Source: CAD feature listing. Evaluate the final solid. Frame: model axes, mm. A direction names the side the tool comes from. Give positions to 0.01 mm unless a question says otherwise; leave off trailing zeros. Order: outer loops, then holes, each group sorted by start corner. A loop starts at its lowest first (then second) coordinate and runs counter-clockwise, first axis right, second up.
```python
from build123d import *

# Parameters (mm, degrees)
PAD_DEPTH    = 0.375
SKETCH002_R  = 1.5
PAD001_DEPTH = 0.5


with BuildPart() as part:
    # Sketch → Pad (new body, symmetric)
    with BuildSketch(Plane.XY):
        with BuildLine():
            Line((-0.25, 0), (0, 0))
            Line((0, 0), (0.25, 0))
            ThreePointArc((0.25, 0), (8.71609, -20.785997), (29.295895, -29.741667))
            ThreePointArc((29.290002, -30.241667), (30.749948, -30.008839), (29.295895, -29.741667))
            ThreePointArc((-0.25, 0), (8.360454, -21.137467), (29.290002, -30.241667))
        make_face()
    extrude(amount=PAD_DEPTH, both=True)

    # Sketch002 → Pad001 (join)
    with BuildSketch(Plane.XZ):
        Circle(SKETCH002_R)
    extrude(amount=PAD001_DEPTH)

    # Sphere → Sphere (revolve, cut)
    with BuildSketch(Plane(origin=(30, -30, 0.6925), x_dir=(1, 0, 0), z_dir=(0, -1, 0))):
        with BuildLine():
            ThreePointArc((0, -0.635), (0.635, 0), (0, 0.635))
            Line((0, 0.635), (0, -0.635))
        make_face()
    revolve(axis=Axis((30, -30, 0.6925), (0, 0, 1)), mode=Mode.SUBTRACT)


solid = part.part
```
1) Section query B-B, the plane y = -24. Return the cut outline in (x, z) (3 decimals).
Report:
outline: (11.586, -0.375) - (12.42, -0.375) - (12.42, 0.375) - (11.586, 0.375) - close
2) Section query C-C, the plane z = 0.75. Return the cut outline in (x, y), and give its area (3 significant figures).
Report:
outline: (-1.3, -0.5) - (1.3, -0.5) - (1.3, 0) - (-1.3, 0) - close
area: 1.30 mm2
3) Reachability of faces 1 (the flat face through (0, 0, 0)), 2 (the flat face through (6, -18, 0.375)) from +Z, -Z, +X, -X, +Y, -Y: full face, straight path, thin tool, end or side. Return the list, or none.
Report:
face 1: +Z, -Z, +X, -X, +Y
face 2: +Z, +X, -X, -Y
4) Material intervals for L1, parallel to X at y = -11, z = 0.2; L2, parallel to Y at x = 16.5, z = 0.1; L3, parallel to X at y = -9.5, z = -0.25, sorted ascending.
Report:
L1: x = 1.82 to 2.36
L2: y = -27.07 to -26.51
L3: x = 1.28 to 1.81
5) Draft query along X for faces 3 (the cylindrical face through (-1.5, -0.25, 0.07)), 4 (the cylindrical face through (8.309, -21.084, 0.005)), 5 (the flat face through (6, -18, -0.375)), 6 (the cylindrical face through (30.75, -30.04, 0.01)). Return one class per face: +X half, -X half, draft (parallel to the pull), parting line (faces both ways), or undercut.
Report:
face 3: parting line
face 4: -X half
face 5: draft
face 6: undercut
6) Pin query (flat end, axial travel): pin 1 (1 mm diameter, centred on y = -12.5, z = 0.5, fed in from -X); pin 2 (1.5 mm diameter, centred on x = 24, z = -1, fed in from +Y); pin 3 (1.5 mm diameter, centred on x = 10, z = 0, fed in from -Y). Return the tip coordinate at first contact, or that it passes through.
Report:
pin 1: stops at x = 2.24
pin 2: stops at y = -29.05
pin 3: stops at y = -23.33
